Drawing for the job (mm, zero at the part's lowest x, y, z). Round coordinates to 2 decimals unless told otherwise and drop trailing zeros. Write each loop counter-clockwise with the first axis right and the second up, starting at its lowest first coordinate (ties: lowest second). Pieces come first, ordered by that corner, then holes.
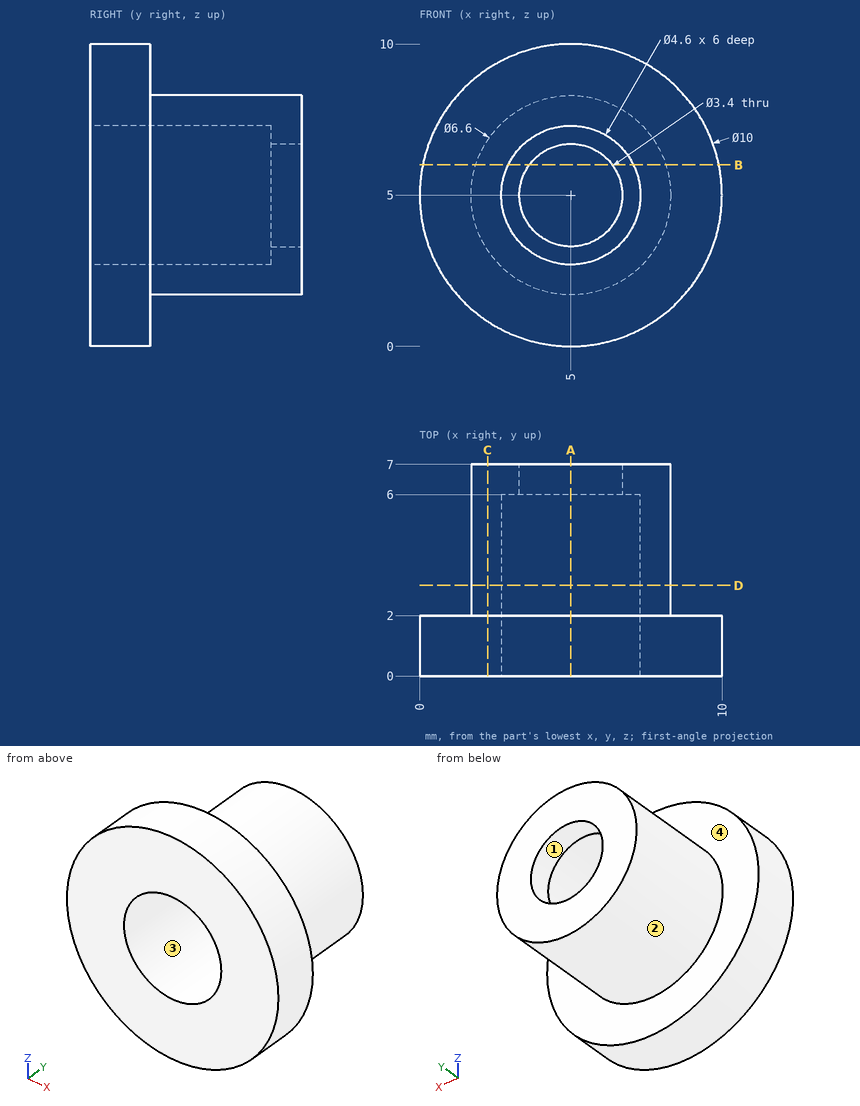
1) Cut at A-A on x = 5. List the corners of the cut face in (y, z).
2) Cut at D-D on y = 3. List the corners of the cut face in (x, z), and give its area (3 significant figures).
3) Cut at B-B on z = 6. List the corners of the cut face in (x, y).
4) Wall check: probe 1 along X at (y, z) = (3.25, 5); probe 2 along X at (y, z) = (6.55, 5). Give the ranges that are in metal, low to high.
5) Flat gauge pins, fed straight in: pin 1 Ø3 at (x, y) = (5.5, 5.5) entering from -Z; pin 2 Ø2 at (y, z) = (4, 5) entering from +X; pin 3 Ø4.5 at (x, z) = (5, 5) entering from -Y. Where does each tip first touch, or does it go through?
6) Pull direction X, two halves, no side cores. Call the marked faces 1, 2, 3 and 4: released by +X, released by -X, zero draft, split by the parting line, or undercut.
7) Cut at C-C on x = 2.25. List the corners of the cut face in (y, z), and give its area (3 significant figures).
Result sheet:
1. outline: (0, 0) - (2, 0) - (2, 1.7) - (7, 1.7) - (7, 3.3) - (6, 3.3) - (6, 2.7) - (0, 2.7) - close; (0, 7.3) - (6, 7.3) - (6, 6.7) - (7, 6.7) - (7, 8.3) - (2, 8.3) - (2, 10) - (0, 10) - close
2. outline: circle Ø6.6 at (5, 5); hole circle Ø4.6 at (5, 5)
2. area: 17.6 mm2
3. outline: (0.1, 0) - (2.93, 0) - (2.93, 6) - (3.63, 6) - (3.63, 7) - (1.86, 7) - (1.86, 2) - (0.1, 2) - close; (6.37, 6) - (7.07, 6) - (7.07, 0) - (9.9, 0) - (9.9, 2) - (8.14, 2) - (8.14, 7) - (6.37, 7) - close
4. probe 1: x = 1.7 to 2.7, 7.3 to 8.3
4. probe 2: x = 1.7 to 3.3, 6.7 to 8.3
5. pin 1: stops at z = 1.7
5. pin 2: stops at x = 8.3
5. pin 3: stops at y = 6
6. face 1: undercut
6. face 2: split by the parting line
6. face 3: undercut
6. face 4: zero draft
7. outline: (0, 0.82) - (2, 0.82) - (2, 3.18) - (7, 3.18) - (7, 6.82) - (2, 6.82) - (2, 9.18) - (0, 9.18) - close
7. area: 34.9 mm2
